Part model, mm, in its own coordinate system. Face numbers are marked on the shaded views. A direction names the side the tool comes from. Give positions to 0.01 mm unless a question says otherwise; leave off trailing zeros. Loops run counter-clockwise (first coordinate to the right, second up) from the corner with the lowest first, then second, coordinate; pieces in that order, holes last. Notation, with made-up numbers: (-7, 34.25) -> (49, 34.25) arc R22 ccw to (49, 67.25) -> close; hole circle Ø6 at (-21.5, 84). An arc over 180 degrees is marked (long way). One line per question, with ' | ' between items.
```python
from build123d import *

# Parameters (mm, degrees)
BOSS_EXTRUDE1_DEPTH = 4
CHAMFER1_SIZE       = 4
SKETCH2_W           = 8
SKETCH2_H           = 4
SKETCH2_W_2         = 12
BOSS_EXTRUDE2_DEPTH = 4


with BuildPart() as part:
    # Sketch1 → Boss-Extrude1 (new body)
    with BuildSketch(Plane.XY):
        Polygon((0, 34), (0, 0), (4, 0), (4, 4), (8, 4), (8, 22), (24.035, 22), (24.035, 28), (26.035, 28), (26.035, 34), align=None)
        Polygon((52.07, 34), (26.035, 34), (26.035, 28), (28.035, 28), (28.035, 22), (44.07, 22), (44.07, 4), (48.07, 4), (48.07, 0), (52.07, 0), align=None)
    extrude(amount=BOSS_EXTRUDE1_DEPTH)

    # Chamfer1
    chamfer1_edges = [part.edges().sort_by_distance(p)[0] for p in [
        (44.07, 22, 2),
        (8, 22, 2),
    ]]
    chamfer(chamfer1_edges, length=CHAMFER1_SIZE)

    # Sketch2 → Boss-Extrude2 (add)
    with BuildSketch(Plane.XY.offset(4)):
        with Locations((4, 36)):
            Rectangle(SKETCH2_W, SKETCH2_H)
        with Locations((48.07, 36)):
            Rectangle(SKETCH2_W, SKETCH2_H)
        with Locations((26.035, 36)):
            Rectangle(SKETCH2_W_2, SKETCH2_H)
    extrude(amount=-BOSS_EXTRUDE2_DEPTH)


solid = part.part
```
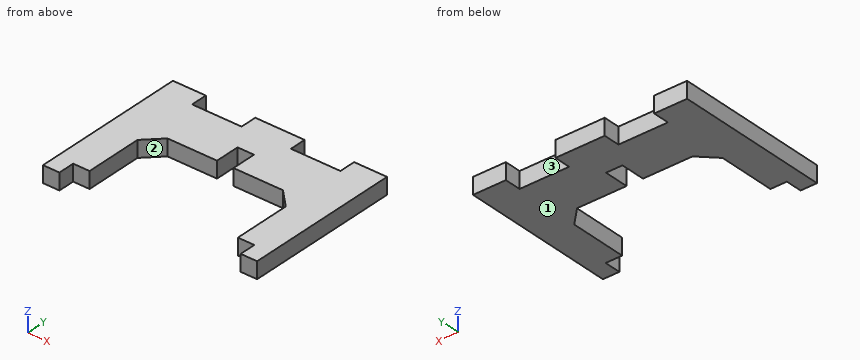
1) Pin check, flat tips, straight feed: P1, Ø2, axis at x = 39, z = 2, coming from the +Y side; P2, Ø2, axis at x = 25.5, z = 1.5, coming from the -Y side; P3, Ø2, axis at x = 6, z = 2, coming from the -Y side. Stop position of each tip, or through.
Found:
P1: y = 34 | P2: y = 28 | P3: y = 4
2) Saw through at A-A (y = 10). Give the cut face in (x, z).
Found:
outline: (0, 0) -> (8, 0) -> (8, 4) -> (0, 4) -> close; (44.07, 0) -> (52.07, 0) -> (52.07, 4) -> (44.07, 4) -> close
3) Saw through at C-C (y = 23.5). Give the cut face in (x, z) (3 decimals).
Found:
outline: (0, 0) -> (24.035, 0) -> (24.035, 4) -> (0, 4) -> close; (28.035, 0) -> (52.07, 0) -> (52.07, 4) -> (28.035, 4) -> close
4) Saw through at D-D (x = 45). Give the cut face in (y, z), and give its area (3 significant figures).
Found:
outline: (4, 0) -> (38, 0) -> (38, 4) -> (4, 4) -> close | area: 136 mm2
5) Saw through at B-B (z = 2.3). Give the cut face in (x, y) (3 decimals), and give its area (3 significant figures).
Found:
outline: (0, 0) -> (4, 0) -> (4, 4) -> (8, 4) -> (8, 18) -> (12, 22) -> (24.035, 22) -> (24.035, 28) -> (28.035, 28) -> (28.035, 22) -> (40.07, 22) -> (44.07, 18) -> (44.07, 4) -> (48.07, 4) -> (48.07, 0) -> (52.07, 0) -> (52.07, 38) -> (44.07, 38) -> (44.07, 34) -> (32.035, 34) -> (32.035, 38) -> (20.035, 38) -> (20.035, 34) -> (8, 34) -> (8, 38) -> (0, 38) -> close | area: 1,050 mm2
6) Drill centre lines: line 1 (X direction, y = 36.5, z = 1.05) (3 decimals); line 2 (X direction, y = 23.5, z = 0.4) (3 decimals); line 3 (X direction, y = 18, z = 2.45). Where is each one in solid material? Low to high.
Found:
line 1: 0 to 8, 20.035 to 32.035, 44.07 to 52.07 | line 2: 0 to 24.035, 28.035 to 52.07 | line 3: 0 to 8, 44.07 to 52.07
7) Tool access for the marked faces 1, 2 and 3: list every direction of +Z, -Z, +X, -X, +Y, -Y with a clear straight run to the whole face (end or side of a thin tool).
Found:
face 1: -Z, +X, -X, +Y, -Y | face 2: +Z, -Z, -Y | face 3: +Z, -Z, +Y
